```python
from build123d import *

# Parameters (mm, degrees)
BOSS_EXTRUDE1_DEPTH = 14
SKETCH2_R           = 1.259114001
CUT_EXTRUDE1_DEPTH  = 14


with BuildPart() as part:
    # Sketch1 → Boss-Extrude1 (new body)
    with BuildSketch(Plane(origin=(0, 0, 0), x_dir=(1, 0, 0), z_dir=(0, 1, 0))):
        Polygon((-7.39, 0), (7.39, 0), (7.39, 11.05), (12.39, 11.05), (12.39, 12.64), (5.8, 12.64), (5.8, 1.59), (-5.8, 1.59), (-5.8, 12.64), (-12.39, 12.64), (-12.39, 11.05), (-7.39, 11.05), align=None)
    extrude(amount=BOSS_EXTRUDE1_DEPTH)

    # Sketch2 → Cut-Extrude1 (cut)
    with BuildSketch(Plane.XY.offset(-11.05)):
        with Locations((-9.89, 7)):
            Circle(SKETCH2_R)
        with Locations((9.89, 7)):
            Circle(SKETCH2_R)
    extrude(amount=-CUT_EXTRUDE1_DEPTH, mode=Mode.SUBTRACT)


solid = part.part
```
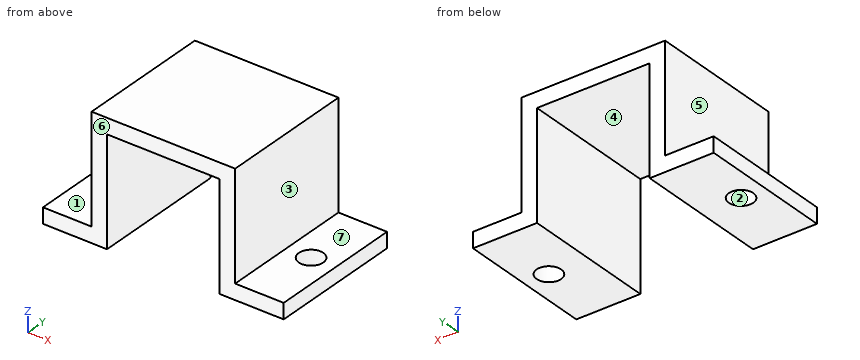
Part model, mm, in its own coordinate system. Face numbers are marked on the shaded views. A direction names the side the tool comes from. Round coordinates to 2 decimals unless told otherwise and drop trailing zeros. Write each loop counter-clockwise with the first axis right and the second up, starting at its lowest first coordinate (ties: lowest second). Pieces come first, ordered by that corner, then holes. Notation, with made-up numbers: (51, -7.5) -> (85, -7.5) arc R14 cw to (85, 11.5) -> close; hole circle Ø1 at (56, -25.75). An arc over 180 degrees is marked (long way). Return JSON: item names as keys, results as strings. Group by question number.
Q1. Which spindle directions (+Z, -Z, +X, -X, +Y, -Y) get a long thin tool onto all of the face, cutting with end or side? Do the marked faces 4, 5, 6 and 7. Say none if no direction does.
Q2. Probe L1, parallel to X at y = 1.75, z = -7.5; L2, parallel to Y at x = 9.89, z = -12.1; L3, parallel to Z at x = -5.75, y = 9. List the from-to ranges inside material, lowest first. Write a range as [from, to].
Q3. Saw through at B-B on x = 9.89. Write the cut outline in (y, z).
Q4. Saw through at A-A on z = -11.5. Write the cut outline in (x, y).
Q5. Pin check, flat tips, straight feed: pin 1 (3.5 mm diameter, centred on y = 9, z = -6.5, fed in from +X); pin 2 (1.5 mm diameter, centred on y = 5, z = -10.5, fed in from -X); pin 3 (5.5 mm diameter, centred on y = 4.5, z = -5.5, fed in from -X); pin 4 (4 mm diameter, centred on x = -9.89, y = 7, fed in from +Z). Stop position of each tip, or through.
Q6. Mould opens along X. For the marked faces 1, 2 and 3 say: pulls with the +X half, pulls with the -X half, needs draft (parallel to the pull), parting line crosses it, or undercut.
Q7. Saw through at D-D on y = 7. Write the cut outline in (x, z).
Q8. Saw through at C-C on z = -5. Write the cut outline in (x, y), plus the area to 3 significant figures.
Answer:
{
 "1": {"face 4": "-Z, +Y, -Y", "face 5": "+Z, -X, +Y, -Y", "face 6": "+Z, -Z, +X, -X, -Y", "face 7": "+Z, +X, +Y, -Y"},
 "2": {"L1": "[-7.39, -5.8], [5.8, 7.39]", "L2": "[0, 5.74], [8.26, 14]", "L3": "[-1.59, 0]"},
 "3": {"outline": "(0, -12.64) -> (5.74, -12.64) -> (5.74, -11.05) -> (0, -11.05) -> close; (8.26, -12.64) -> (14, -12.64) -> (14, -11.05) -> (8.26, -11.05) -> close"},
 "4": {"outline": "(-12.39, 0) -> (-5.8, 0) -> (-5.8, 14) -> (-12.39, 14) -> close; (5.8, 0) -> (12.39, 0) -> (12.39, 14) -> (5.8, 14) -> close; hole circle Ø2.52 at (-9.89, 7); hole circle Ø2.52 at (9.89, 7)"},
 "5": {"pin 1": "x = 7.39", "pin 2": "x = -12.39", "pin 3": "x = -7.39", "pin 4": "z = -11.05"},
 "6": {"face 1": "needs draft", "face 2": "undercut", "face 3": "pulls with the +X half"},
 "7": {"outline": "(-12.39, -12.64) -> (-11.15, -12.64) -> (-11.15, -11.05) -> (-12.39, -11.05) -> close; (-8.63, -12.64) -> (-5.8, -12.64) -> (-5.8, -1.59) -> (5.8, -1.59) -> (5.8, -12.64) -> (8.63, -12.64) -> (8.63, -11.05) -> (7.39, -11.05) -> (7.39, 0) -> (-7.39, 0) -> (-7.39, -11.05) -> (-8.63, -11.05) -> close; (11.15, -12.64) -> (12.39, -12.64) -> (12.39, -11.05) -> (11.15, -11.05) -> close"},
 "8": {"outline": "(-7.39, 0) -> (-5.8, 0) -> (-5.8, 14) -> (-7.39, 14) -> close; (5.8, 0) -> (7.39, 0) -> (7.39, 14) -> (5.8, 14) -> close", "area": "44.5 mm2"}
}
